Answer from the drawing. Dimensions are ordinates in mm from the lowest x, y and z of the part. A direction names the side the tool comes from. Give positions to 0.01 mm unless a question says otherwise; leave off trailing zeros. Loops run counter-clockwise (first coordinate to the right, second up) from the corner with the lowest first, then second, coordinate; pieces in that order, holes last. Notation, with made-up numbers: M 62.5,-22.5 L 116.5,-22.5 A12 cw 116.5,0.5 Z; hole C 22,67.5 d7. An arc over 180 degrees is marked long. Use a Markdown table: item, result.
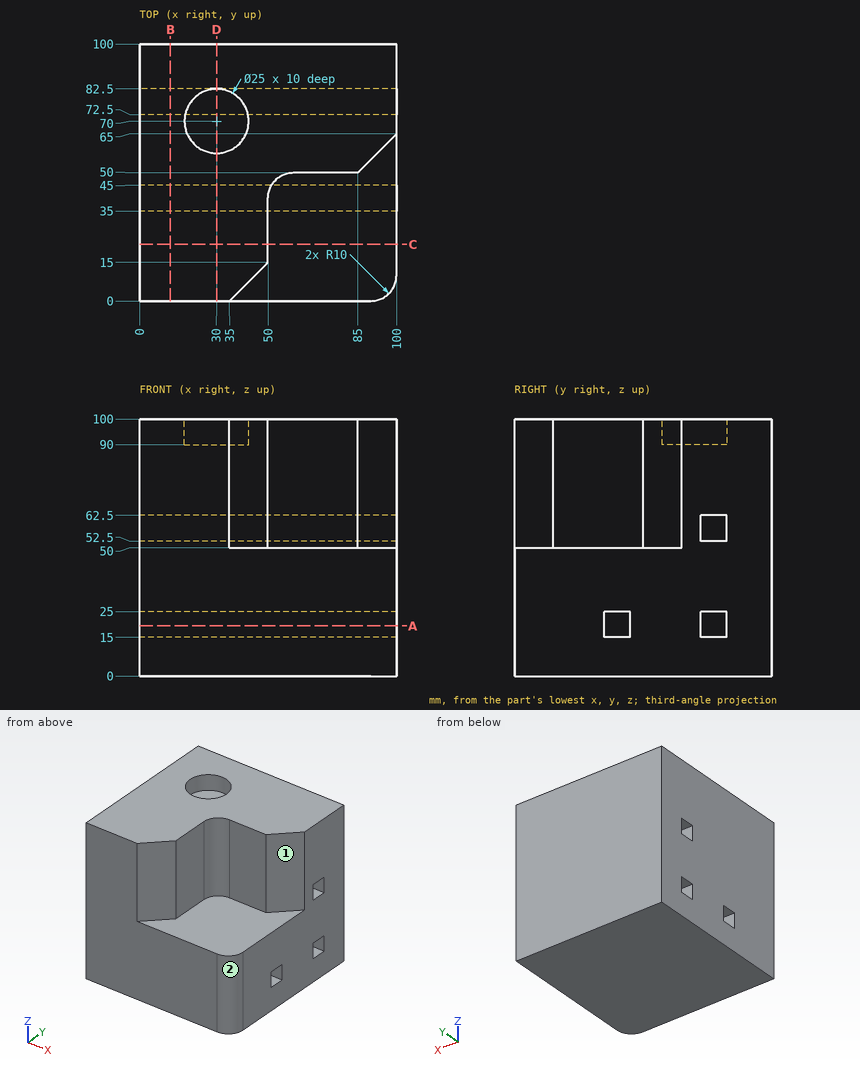
(1) Which of the six approach directions +Z, -Z, +X, -X, +Y, -Y give full straight-line access (tool end or side, diameter ignored) to the marked faces 1 and 2?
Entries:
| item | result |
|---|---|
| face 1 | +Z, +X, -Y |
| face 2 | +Z, -Z, +X, -Y |
(2) A cutting plane is placed at C-C (y = 22). Write down the section's boundary in (x, z), and give its area (3 significant figures).
Entries:
| item | result |
|---|---|
| outline | M 0,0 L 100,0 L 100,50 L 50,50 L 50,100 L 0,100 Z |
| area | 7,500 mm² |
(3) Consider probe 1 along Z at (x, y) = (48, 80); probe 2 along Y at (x, z) = (30, 94.5); probe 3 along Z at (x, y) = (34, 81). Determine where each line is inside the solid, lowest interval first. Write a range as [from, to].
Entries:
| item | result |
|---|---|
| probe 1 | z = [0, 15], [25, 52.5], [62.5, 100] |
| probe 2 | y = [0, 57.5], [82.5, 100] |
| probe 3 | z = [0, 15], [25, 52.5], [62.5, 90] |
(4) A cutting plane is placed at D-D (x = 30). Write down the section's boundary in (y, z), and give its area (3 significant figures).
Entries:
| item | result |
|---|---|
| outline | M 0,0 L 100,0 L 100,100 L 82.5,100 L 82.5,90 L 57.5,90 L 57.5,100 L 0,100 Z; hole M 35,15 L 45,15 L 45,25 L 35,25 Z; hole M 72.5,15 L 82.5,15 L 82.5,25 L 72.5,25 Z; hole M 72.5,52.5 L 82.5,52.5 L 82.5,62.5 L 72.5,62.5 Z |
| area | 9,450 mm² |
(5) Given P1, Ø1.5, axis at y = 20.5, z = 84.5, coming from the +X side; P2, Ø8, axis at x = 80, y = 32.5, coming from the +Z side; P3, Ø12.5, axis at x = 30, y = 66, coming from the +Z side, each flat-ended and moving along its own axis, determine where each tip first touches the part or whether it passes through.
Entries:
| item | result |
|---|---|
| P1 | stops at x = 50 |
| P2 | stops at z = 50 |
| P3 | stops at z = 90 |
(6) A cutting plane is placed at A-A (z = 19.5). Write down the section's boundary in (x, y).
Entries:
| item | result |
|---|---|
| outline | M 0,0 L 90,0 A10 ccw 100,10 L 100,35 L 0,35 Z; M 0,45 L 100,45 L 100,72.5 L 0,72.5 Z; M 0,82.5 L 100,82.5 L 100,100 L 0,100 Z |
(7) A cutting plane is placed at B-B (x = 12). Write down the section's boundary in (y, z).
Entries:
| item | result |
|---|---|
| outline | M 0,0 L 100,0 L 100,100 L 0,100 Z; hole M 35,15 L 45,15 L 45,25 L 35,25 Z; hole M 72.5,15 L 82.5,15 L 82.5,25 L 72.5,25 Z; hole M 72.5,52.5 L 82.5,52.5 L 82.5,62.5 L 72.5,62.5 Z |
